Part model, mm, in its own coordinate system. A direction names the side the tool comes from. Round coordinates to 2 decimals unless told otherwise and drop trailing zeros. Loops run counter-clockwise (first coordinate to the right, second up) from the corner with the lowest first, then second, coordinate; pieces in that order, holes last.
from build123d import *

# Parameters (mm, degrees)
SKETCH_2_W            = 80
SKETCH_2_H            = 20
EXTRUDE_1_DEPTH       = 3
EXTRUDE_2_DEPTH       = 20
HOLE_WIZARD_3_0_3_1_D = 3
HOLE_WIZARD_4_0_4_1_D = 4
CUT_EXTRUDE_1_DEPTH   = 200
FILLET_1_R            = 5


with BuildPart() as part:
    # 草图2 → 凸台-拉伸1 (new body)
    with BuildSketch(Plane(origin=(0, 0, 0), x_dir=(1, 0, 0), z_dir=(0, 1, 0))):
        Rectangle(SKETCH_2_W, SKETCH_2_H)
    extrude(amount=EXTRUDE_1_DEPTH)

    # 草图3 → 凸台-拉伸2 (add)
    with BuildSketch(Plane.XY.offset(10)):
        Polygon((-9, 13), (-19, 3), (-5, 3), (-5, 33), (-9, 33), align=None)
    extrude_2 = extrude(amount=-EXTRUDE_2_DEPTH)

    # 镜向1: 凸台-拉伸2 across plane
    add(extrude_2.mirror(Plane.ZY))

    # Ø3.0 (3) 直径孔1 (through all)
    with Locations(Plane.ZY.offset(9)):
        with Locations((0, 28), (0, 18)):
            Hole(HOLE_WIZARD_3_0_3_1_D / 2)

    # Ø4.0 (4) 直径孔1 (through all)
    with Locations(Plane(origin=(0, 3, 0), x_dir=(1, 0, 0), z_dir=(0, 1, 0))):
        with Locations((-30, 0), (30, 0)):
            Hole(HOLE_WIZARD_4_0_4_1_D / 2)

    # 草图10 → 切除-拉伸1 (cut)
    with BuildSketch(Plane.ZY.offset(9)):
        Polygon((10, 13), (10, 33), (5, 33), align=None)
        Polygon((-10, 13), (-10, 33), (-5, 33), align=None)
    extrude(amount=-CUT_EXTRUDE_1_DEPTH, mode=Mode.SUBTRACT)

    # 圆角1
    fillet_1_edges = [part.edges().sort_by_distance(p)[0] for p in [
        (40, 1.5, -10),
        (40, 1.5, 10),
        (-40, 1.5, 10),
        (-40, 1.5, -10),
    ]]
    fillet(fillet_1_edges, radius=FILLET_1_R)


solid = part.part
1) Drop flat-ended pins along their axis: pin 1 Ø10 at (y, z) = (23.5, -4.5) entering from +X; pin 2 Ø6 at (y, z) = (23.5, -3.5) entering from -X; pin 3 Ø8 at (x, z) = (9.5, 3) entering from +Y; pin 4 Ø6 at (y, z) = (15.5, -2.5) entering from -X. Give the stop position or say it passes through.
Values:
pin 1: stops at x = 9
pin 2: stops at x = -9
pin 3: stops at y = 33
pin 4: stops at x = -9.5
2) Slice it at D-D, the plane z = -3.75. Give the cut face in (x, y), then the cut area to 3 significant figures.
Values:
outline: (-40, 0) - (40, 0) - (40, 3) - (19, 3) - (9, 13) - (9, 33) - (5, 33) - (5, 3) - (-5, 3) - (-5, 33) - (-9, 33) - (-9, 13) - (-19, 3) - (-40, 3) - close
area: 580 mm2
3) Tool access for faces 5 (the face through (-6.972, 19.487, 0.195)), 6 (the face through (27, 3, 0)), 7 (the face through (-5, 14, 0)): list every direction of +Z, -Z, +X, -X, +Y, -Y with a clear straight run to the whole face (end or side of a thin tool).
Values:
face 5: +X, -X
face 6: +Z, -Z, +X, +Y
face 7: +Z, -Z, +Y
4) Wall check: line 1 along Y through (x, z) = (-5.9, 0); line 2 along X through (y, z) = (26.5, -0.75); line 3 along Z through (x, y) = (-30, 1.5). Give the ranges that are in metal, low to high.
Values:
line 1: y = 0 to 16.5, 19.5 to 26.5, 29.5 to 33
line 2: x = -9 to -5, 5 to 9
line 3: z = -10 to -2, 2 to 10
5) Mould opens along Z. For faces 1 (the face through (-31.908, 1.479, -0.601)), 2 (the face through (7.028, 29.487, 0.195)), 3 (the face through (6.972, 23.14, 7.465)), 4 (the face through (-9, 21, 0)) say: released by +Z, released by -Z, zero draft, split by the parting line, or undercut.
Values:
face 1: undercut
face 2: undercut
face 3: released by +Z
face 4: zero draft
6) Slice it at C-C, the plane z = 0. Give the number of separate pieces and of enclosed holes in the cut face, then the cut area to 3 significant figures.
Values:
separate pieces: 7
enclosed holes: 0
area: 508 mm2
7) Slice it at B-B, the plane y = 28. Give the cut face in (x, z).
Values:
outline: (-9, -6.25) - (-5, -6.25) - (-5, -1.5) - (-9, -1.5) - close; (-9, 1.5) - (-5, 1.5) - (-5, 6.25) - (-9, 6.25) - close; (5, -6.25) - (9, -6.25) - (9, -1.5) - (5, -1.5) - close; (5, 1.5) - (9, 1.5) - (9, 6.25) - (5, 6.25) - close
8) Slice it at A-A, the plane x = 30. Give the cut face in (y, z), then the cut area to 3 significant figures.
Values:
outline: (0, -10) - (3, -10) - (3, -2) - (0, -2) - close; (0, 2) - (3, 2) - (3, 10) - (0, 10) - close
area: 48.0 mm2
